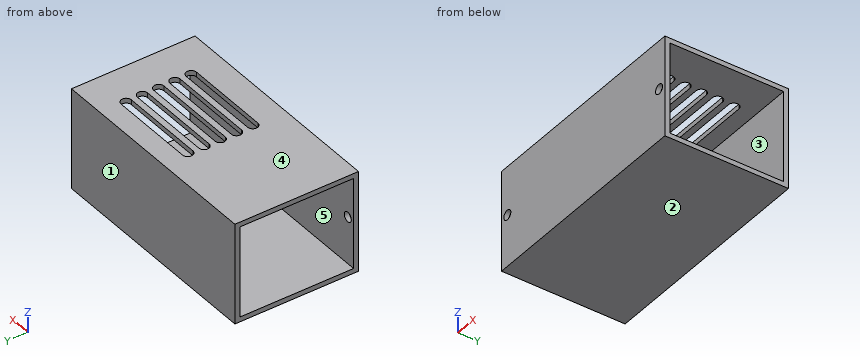
from build123d import *

# Parameters (mm, degrees)
SKETCH_1_W          = 70
SKETCH_1_H          = 38
EXTRUDE_1_DEPTH     = 31
SKETCH_2_W          = 28
SKETCH_2_H          = 35
CUT_EXTRUDE_1_DEPTH = 71
CUT_EXTRUDE_3_DEPTH = 2
SKETCH_5_R          = 1.5
CUT_EXTRUDE_4_DEPTH = 2


with BuildPart() as part:
    # 草图1 → 凸台-拉伸1 (new body)
    with BuildSketch(Plane.XY):
        Rectangle(SKETCH_1_W, SKETCH_1_H)
    extrude(amount=EXTRUDE_1_DEPTH)

    # 草图2 → 切除-拉伸1 (cut, through all)
    with BuildSketch(Plane(origin=(35, 0, 0), x_dir=(0, 0, -1), z_dir=(1, 0, 0))):
        with Locations((-15.5, 0)):
            Rectangle(SKETCH_2_W, SKETCH_2_H)
    extrude(amount=-CUT_EXTRUDE_1_DEPTH, mode=Mode.SUBTRACT)

    # 草图4 → 切除-拉伸3 (cut)
    with BuildSketch(Plane.XY.offset(31)):
        with BuildLine():
            Line((-3.793519022, 12.68225477), (22.537965955, 12.68225477))
            ThreePointArc((22.537965955, 12.68225477), (24.1000032, 11.120217526), (22.537965955, 9.558180281))
            Line((22.537965955, 9.558180281), (-3.793519022, 9.558180281))
            ThreePointArc((-3.793519022, 9.558180281), (-5.355556267, 11.120217526), (-3.793519022, 12.68225477))
        make_face()
        with BuildLine():
            Line((-3.793519022, 4.558180281), (22.537965955, 4.558180281))
            ThreePointArc((22.537965955, 4.558180281), (24.1000032, 6.120217526), (22.537965955, 7.68225477))
            Line((22.537965955, 7.68225477), (-3.793519022, 7.68225477))
            ThreePointArc((-3.793519022, 7.68225477), (-5.355556267, 6.120217526), (-3.793519022, 4.558180281))
        make_face()
        with BuildLine():
            Line((-3.793519022, -0.441819719), (22.537965955, -0.441819719))
            ThreePointArc((22.537965955, -0.441819719), (24.1000032, 1.120217526), (22.537965955, 2.68225477))
            Line((22.537965955, 2.68225477), (-3.793519022, 2.68225477))
            ThreePointArc((-3.793519022, 2.68225477), (-5.355556267, 1.120217526), (-3.793519022, -0.441819719))
        make_face()
        with BuildLine():
            Line((-3.793519022, -5.441819719), (22.537965955, -5.441819719))
            ThreePointArc((22.537965955, -5.441819719), (24.1000032, -3.879782474), (22.537965955, -2.31774523))
            Line((22.537965955, -2.31774523), (-3.793519022, -2.31774523))
            ThreePointArc((-3.793519022, -2.31774523), (-5.355556267, -3.879782474), (-3.793519022, -5.441819719))
        make_face()
        with BuildLine():
            Line((-3.793519022, -10.441819719), (22.537965955, -10.441819719))
            ThreePointArc((22.537965955, -10.441819719), (24.1000032, -8.879782474), (22.537965955, -7.31774523))
            Line((22.537965955, -7.31774523), (-3.793519022, -7.31774523))
            ThreePointArc((-3.793519022, -7.31774523), (-5.355556267, -8.879782474), (-3.793519022, -10.441819719))
        make_face()
    extrude(amount=-CUT_EXTRUDE_3_DEPTH, mode=Mode.SUBTRACT)

    # 草图5 → 切除-拉伸4 (cut)
    with BuildSketch(Plane.XZ.offset(19)):
        with Locations((-32.5, 16)):
            Circle(SKETCH_5_R)
        with Locations((32.5, 16)):
            Circle(SKETCH_5_R)
    extrude(amount=-CUT_EXTRUDE_4_DEPTH, mode=Mode.SUBTRACT)


solid = part.part
Read the model definition and answer for the solid it produces. Units are mm, in the model's axes. Face numbers are marked on the shaded views. A direction names the side the tool comes from. Coordinates: 2 decimals unless noted, no trailing zeros. Order: outer loops, then holes, each group sorted by start corner. A loop starts at its lowest first (then second) coordinate and runs counter-clockwise, first axis right, second up. Notation, with made-up numbers: (72.5, 67) -> (126.5, 67) arc R11 cw to (126.5, 80) -> close; hole circle Ø4 at (38.5, 26). An arc over 180 degrees is marked (long way). Answer as a JSON object with one key per item and string values.
1) This flat-tipped pin is pushed along its axis until it touches: pin 1 (12 mm diameter, centred on y = 1, z = 10.5, fed in from -X). Where does it stop, or does it pass through?
Model answer:
{"pin 1": "passes through"}
2) A cutting plane is placed at C-C, the plane x = -26. Determine the outline of the cut face in (y, z), plus the area to 3 significant figures.
Model answer:
{"outline": "(-19, 0) -> (19, 0) -> (19, 31) -> (-19, 31) -> close; hole (-17.5, 1.5) -> (17.5, 1.5) -> (17.5, 29.5) -> (-17.5, 29.5) -> close", "area": "198 mm²"}
3) A tool of negligible diameter and unlimited length cuts with its end or side. For the marked faces 4 and 5, from which of +Z, -Z, +X, -X, +Y, -Y can it reach the whole face along a straight path? Write none if from no direction.
Model answer:
{"face 4": "+Z, +X, -X, +Y, -Y", "face 5": "+X, -X"}
4) A cutting plane is placed at D-D, the plane z = 16. Determine the outline of the cut face in (x, y).
Model answer:
{"outline": "(-35, -19) -> (-34, -19) -> (-34, -17.5) -> (-35, -17.5) -> close; (-35, 17.5) -> (35, 17.5) -> (35, 19) -> (-35, 19) -> close; (-31, -19) -> (31, -19) -> (31, -17.5) -> (-31, -17.5) -> close; (34, -19) -> (35, -19) -> (35, -17.5) -> (34, -17.5) -> close"}
5) A cutting plane is placed at B-B, the plane y = 3.5. Determine the outline of the cut face in (x, z), plus the area to 3 significant figures.
Model answer:
{"outline": "(-35, 0) -> (35, 0) -> (35, 1.5) -> (-35, 1.5) -> close; (-35, 29.5) -> (35, 29.5) -> (35, 31) -> (-35, 31) -> close", "area": "210 mm²"}
6) Consider line 1 along Y through (x, z) = (5, 30); line 2 along Y through (x, z) = (18, 20); line 3 along Z through (x, y) = (10, -10.5). Determine where each line is inside the solid, lowest interval first. Write a range as from..to.
Model answer:
{"line 1": "y = -19..-10.44, -7.32..-5.44, -2.32..-0.44, 2.68..4.56, 7.68..9.56, 12.68..19", "line 2": "y = -19..-17.5, 17.5..19", "line 3": "z = 0..1.5, 29.5..31"}
7) The mould has two halves that part along Y. Classify the marked faces 1, 2 and 3: released by +Y, released by -Y, zero draft, split by the parting line, or undercut.
Model answer:
{"face 1": "released by +Y", "face 2": "zero draft", "face 3": "undercut"}
8) A cutting plane is placed at A-A, the plane z = 23. Determine the outline of the cut face in (x, y).
Model answer:
{"outline": "(-35, -19) -> (35, -19) -> (35, -17.5) -> (-35, -17.5) -> close; (-35, 17.5) -> (35, 17.5) -> (35, 19) -> (-35, 19) -> close"}
